from build123d import *

# Parameters (mm, degrees)
F2_SIZE = 1.5
F3_SIZE = 1.5


with BuildPart() as f1:
    # F0 (on Top) → F1 (revolve)
    with BuildSketch(Plane.XY):
        Polygon((3, 5), (0, 5), (0, 10), (-23, 10), (-23, 2.5), (-22, 2.5), (-13, 2.5), (-13, 0), (0, 0), (18.471096, 0), (3, 8), align=None)
    revolve(axis=Axis((9.235548, 0, 0), (-1, 0, 0)))

    # F2
    f2_edges = [f1.edges().sort_by_distance(p)[0] for p in [
        (0, -10, 0),
        (-23, -10, 0),
        (-11.5, 10, 0),
    ]]
    chamfer(f2_edges, length=F2_SIZE)

    # F3
    f3_edges = [f1.edges().sort_by_distance(p)[0] for p in [
        (3, -8, 0),
    ]]
    chamfer(f3_edges, length=F3_SIZE)


solid = f1.part
Geometry check sheet. Reference: the model listing, model coordinates, mm. A direction names the side the tool comes from. Coordinates: 2 decimals unless noted, no trailing zeros. Order: outer loops, then holes, each group sorted by start corner. A loop starts at its lowest first (then second) coordinate and runs counter-clockwise, first axis right, second up. Notation, with made-up numbers: (-11, 74.25) -> (3, 74.25) arc R23 ccw to (3, 112.25) -> close; hole circle Ø1 at (50.25, 84). An arc over 180 degrees is marked (long way). Use a Markdown table: item, result. Add a question column.
1. Material ranges on L1, parallel to Y at x = -20.25, z = 0; L2, parallel to X at y = 6.75, z = 0.75, recorded low to high.
2. Go/stop test with flat-tipped pins: pin 1 Ø8 at (x, z) = (3.5, 4) entering from -Y; pin 2 Ø3 at (x, y) = (-8.5, -1) entering from -Z; pin 3 Ø8 at (x, z) = (-4.5, 6) entering from +Y; pin 4 Ø3 at (x, z) = (11, -2) entering from -Y. Record where each tip stops, or that it passes through.
3. Cross-section at B-B (x = -8). Enter the section's corners in (y, z).
4. Set-up check for faces 5 (the face through (-23, 2, 2)), 6 (the face through (0, -4, 4)), 7 (the face through (-17.93, -0.54, 2.44)): record each of +Z, -Z, +X, -X, +Y, -Y from which the full face is reachable in a straight line by a thin tool's end or side.
5. Mould release check, pull along X, two halves, no side actions. Record for faces 1 (the face through (-13, 0, 0)), 2 (the face through (-11.64, -2.17, 9.76)), 3 (the face through (1.48, -1.08, 4.88)), 4 (the face through (12.874, -0.627, 2.826)): pulls with the +X half, pulls with the -X half, needs draft (parallel to the pull), parting line crosses it, or undercut.
6. Cross-section at A-A (x = -13.5). Enter the section's corners in (y, z).
Filled sheet:
| question | item | result |
|---|---|---|
| 1 | L1 | -10 to -2.5, 2.5 to 10 |
| 1 | L2 | -23 to 0, 3.48 to 5.34 |
| 2 | pin 1 | y = -8.36 |
| 2 | pin 2 | z = -10 |
| 2 | pin 3 | y = 9.8 |
| 2 | pin 4 | y = -4.36 |
| 3 | outline | circle Ø20 at (0, 0) |
| 4 | face 5 | +Z, -Z, -X, +Y, -Y |
| 4 | face 6 | none |
| 4 | face 7 | -X |
| 5 | face 1 | pulls with the -X half |
| 5 | face 2 | needs draft |
| 5 | face 3 | undercut |
| 5 | face 4 | pulls with the +X half |
| 6 | outline | circle Ø20 at (0, 0); hole circle Ø5 at (0, 0) |
